Source: CAD feature listing. Evaluate the final solid. Frame: model axes, mm. Face numbers are marked on the shaded views. Round coordinates to 2 decimals unless told otherwise and drop trailing zeros. Loops run counter-clockwise (first coordinate to the right, second up) from the corner with the lowest first, then second, coordinate; pieces in that order, holes last.
(1) Mould query, pull axis Y, two halves, no side actions, for the marked faces 1, 2, 3 and 4. Classes: pulls with the +Y half, pulls with the -Y half, needs draft (parallel to the pull), parting line crosses it, or undercut.
(2) First-contact query: pin 1 Ø2 at (y, z) = (6, 30.5) entering from -X; pin 2 Ø10 at (y, z) = (-12.5, 13) entering from +X; pin 3 Ø4 at (x, z) = (16, 23.5) entering from -Y; pin 4 Ø17 at (x, y) = (0, 0) entering from +Z. Flat tips, straight axial feed; report the tip coordinate or a pass-through.
(3) Section C-C, the plane x = 66.5. Return the cut outline in (y, z).
(4) Section D-D, the plane x = 43. Return the cut outline in (y, z).
(5) Section A-A, the plane z = 9. Count the separate pieces of the cut face and the enclosed holes in it, plus the area to 3 significant figures.
(6) Material intervals for probe 1 along X at (y, z) = (0, 25) (1 decimal); probe 2 along Y at (x, z) = (0, 23) (1 decimal); probe 3 along Z at (x, y) = (68, 3.5), sorted ascending.
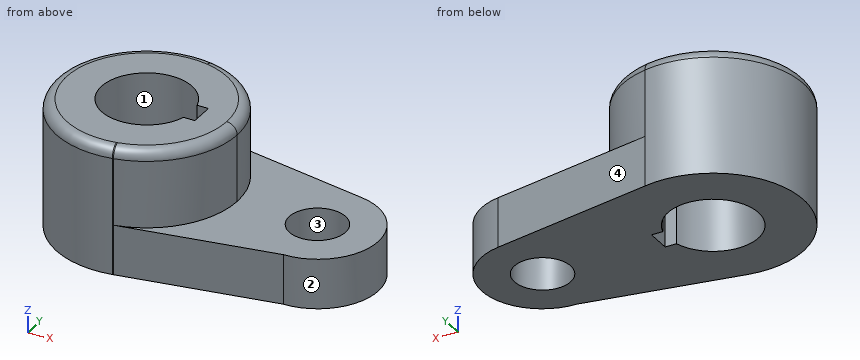
```python
from build123d import *

# Parameters (mm, degrees)
F0_R     = 14.2875
F0_R_2   = 8.89
F1_DEPTH = 15.7734
F2_DEPTH = 40.2336
F4_DEPTH = 40.2346
F5_R     = 3.302


with BuildPart() as f1:
    # F0 (on Top) → F1 (new body)
    with BuildSketch(Plane.XY):
        with BuildLine():
            ThreePointArc((5.362369, -28.067341), (22.019995, -18.211273), (28.575, 0))
            ThreePointArc((28.575, 0), (22.13622, 18.06982), (5.721568, 27.996326))
            ThreePointArc((5.721568, 27.996326), (-28.572841, 0.351263), (5.031592, -28.128521))
            Line((5.031592, -28.128521), (5.362369, -28.067341))
        make_face()
        Circle(F0_R, mode=Mode.SUBTRACT)
        with BuildLine():
            ThreePointArc((5.721568, 27.996326), (22.13622, 18.06982), (28.575, 0))
            ThreePointArc((28.575, 0), (22.019995, -18.211273), (5.362369, -28.067341))
            Line((5.362369, -28.067341), (53.975, -19.075971))
            ThreePointArc((53.975, -19.075971), (73.116672, -1.798756), (57.506479, 18.725075))
            Line((57.506479, 18.725075), (5.721568, 27.996326))
        make_face()
        with Locations((53.975, 0)):
            Circle(F0_R_2, mode=Mode.SUBTRACT)
    extrude(amount=F1_DEPTH)

    # F0 (on Top) → F2 (join)
    with BuildSketch(Plane.XY):
        with BuildLine():
            ThreePointArc((5.362369, -28.067341), (22.019995, -18.211273), (28.575, 0))
            ThreePointArc((28.575, 0), (22.13622, 18.06982), (5.721568, 27.996326))
            ThreePointArc((5.721568, 27.996326), (-28.572841, 0.351263), (5.031592, -28.128521))
            Line((5.031592, -28.128521), (5.362369, -28.067341))
        make_face()
        Circle(F0_R, mode=Mode.SUBTRACT)
    extrude(amount=F2_DEPTH)

    # F3 (on face) → F4 (cut, through all)
    with BuildSketch(Plane.XY):
        with BuildLine():
            Line((17.348139, 3.81), (13.770133, 3.81))
            ThreePointArc((13.770133, 3.81), (14.157567, 1.922483), (14.2875, 0))
            ThreePointArc((14.2875, 0), (14.157567, -1.922483), (13.770133, -3.81))
            Line((13.770133, -3.81), (17.348139, -3.81))
            Line((17.348139, -3.81), (17.348139, 3.81))
        make_face()
    extrude(amount=F4_DEPTH, mode=Mode.SUBTRACT)

    # F5
    f5_edges = [f1.edges().sort_by_distance(p)[0] for p in [
        (-5.19707, 28.098418, 40.2336),
    ]]
    fillet(f5_edges, radius=F5_R)


solid = f1.part
```
Output values:
1. face 1: undercut
1. face 2: parting line crosses it
1. face 3: undercut
1. face 4: pulls with the +Y half
2. pin 1: stops at x = -28.13
2. pin 2: stops at x = 71.67
2. pin 3: stops at y = -24.91
2. pin 4: passes through
3. outline: (-14.53, 0) - (14.48, 0) - (14.48, 15.77) - (-14.53, 15.77) - close
4. outline: (-21.11, 0) - (21.32, 0) - (21.32, 15.77) - (-21.11, 15.77) - close
5. separate pieces: 1
5. enclosed holes: 2
5. area: 3,550 mm2
6. probe 1: x = -28.6 to -14.3, 17.3 to 28.6
6. probe 2: y = -28.6 to -14.3, 14.3 to 28.6
6. probe 3: z = 0 to 15.77
